Read the model definition and answer for the solid it produces. Units are mm, in the model's axes. A direction names the side the tool comes from. Coordinates: 2 decimals unless noted, no trailing zeros. Loops run counter-clockwise (first coordinate to the right, second up) from the corner with the lowest first, then second, coordinate; pieces in that order, holes last. Notation, with made-up numbers: M 82,-28 L 124,-28 A31 cw 124,10 Z; hole C -40,37 d1. An arc over 180 degrees is marked long. Put each result on its own line as item: value.
from build123d import *

# Parameters (mm, degrees)
F0_R     = 7
F1_DEPTH = 20
F2_R     = 8
F3_DEPTH = 12
F5_DEPTH = 25
F8_DEPTH = 6


with BuildPart() as f1:
    # F0 (on Front) → F1 (new body)
    with BuildSketch(Plane.XZ):
        with BuildLine():
            Line((-35, 54), (-35, 0))
            Line((-35, 0), (35, 0))
            Line((35, 0), (35, 54))
            ThreePointArc((35, 54), (33.242641, 58.242641), (29, 60))
            Line((29, 60), (-29, 60))
            ThreePointArc((-29, 60), (-33.242641, 58.242641), (-35, 54))
        make_face()
        with Locations((-21, 46)):
            Circle(F0_R, mode=Mode.SUBTRACT)
        with Locations((21, 46)):
            Circle(F0_R, mode=Mode.SUBTRACT)
    extrude(amount=F1_DEPTH)

    # F2 (on face) → F3 (join)
    with BuildSketch(Plane(origin=(0, 0, 0), x_dir=(1, 0, 0), z_dir=(0, 0, -1))):
        with BuildLine():
            Line((22, 0), (-22, 0))
            ThreePointArc((-22, 0), (-17.757359, -1.757359), (-16, -6))
            Line((-16, -6), (-16, -80))
            ThreePointArc((-16, -80), (0, -96), (16, -80))
            Line((16, -80), (16, -6))
            ThreePointArc((16, -6), (17.757359, -1.757359), (22, 0))
        make_face()
        with Locations((0, -80)):
            Circle(F2_R, mode=Mode.SUBTRACT)
    extrude(amount=-F3_DEPTH)

    # F7 (on Right) → F8 (join, symmetric)
    with BuildSketch(Plane.YZ):
        with BuildLine():
            Line((0, 12), (30, 12))
            ThreePointArc((30, 12), (8.786797, 20.786797), (0, 42))
            Line((0, 42), (0, 12))
        make_face()
    extrude(amount=F8_DEPTH, both=True)


with BuildPart() as f5:
    # F4 (on Right) → F5 (new body)
    with BuildSketch(Plane.YZ):
        Polygon((8.827168, -95.900685), (44.855885, -95.900685), (44.855885, -23.484161), (8.827168, -23.484161), (8.827168, -49.02795), (8.827168, -76.342739), align=None)
    extrude(amount=F5_DEPTH)


solid = f1.part
1) Find section A-A, the plane z = 46. Write down the section's boundary in (x, y), plus the area to 3 significant figures.
Answer list:
outline: M -35,-20 L -28,-20 L -28,0 L -35,0 Z; M -14,-20 L 14,-20 L 14,0 L -14,0 Z; M 28,-20 L 35,-20 L 35,0 L 28,0 Z
area: 840 mm^2
2) Straight lines are drawn through the part: line 1 (X direction, y = 80, z = 3); line 2 (Z direction, x = 21, y = -9); line 3 (Z direction, x = -8, y = 41.5). For each, find the intervals that lie inside material, in ascending order. Write a range as [from, to].
Answer list:
line 1: x = [-16, -8], [8, 16]
line 2: z = [0, 39], [53, 60]
line 3: z = [0, 12]
3) Given pin 1 Ø2 at (x, y) = (-1, 47.5) entering from +Z; pin 2 Ø18 at (x, z) = (-21, 46) entering from +Y; pin 3 Ø10 at (x, z) = (7, 16.5) entering from +Y; pin 4 Ø12 at (x, y) = (18.5, -2) entering from -Z, each flat-ended and moving along its own axis, determine where each tip first touches the part or whether it passes through.
Answer list:
pin 1: stops at z = 12
pin 2: stops at y = 0
pin 3: stops at y = 95.26
pin 4: stops at z = 0
4) Find section B-B, the plane x = 0. Write down the section's boundary in (y, z).
Answer list:
outline: M -20,0 L 72,0 L 72,12 L 30,12 A30 cw 0,42 L 0,60 L -20,60 Z; M 88,0 L 96,0 L 96,12 L 88,12 Z
5) Find section C-C, the plane y = -13. Write down the section's boundary in (x, z), plus the area to 3 significant figures.
Answer list:
outline: M -35,0 L 35,0 L 35,54 A6 ccw 29,60 L -29,60 A6 ccw -35,54 Z; hole C -21,46 d14; hole C 21,46 d14
area: 3,880 mm^2
6) Determine the mould class of faces 6 (the cylindrical face through (-1.041, 72.068, 5.916)), 7 (the cylindrical face through (33.289, -9.86, 58.196)), 8 (the cylindrical face through (0, 96, 6)) for opening direction Y: released by +Y, released by -Y, zero draft, split by the parting line, or undercut.
Answer list:
face 6: undercut
face 7: zero draft
face 8: released by +Y
7) Find section D-D, the plane z = 18. Write down the section's boundary in (x, y), plus the area to 3 significant figures.
Answer list:
outline: M -35,-20 L 35,-20 L 35,0 L 6,0 L 6,12 L -6,12 L -6,0 L -35,0 Z
area: 1,540 mm^2
8) Which of the six approach directions +Z, -Z, +X, -X, +Y, -Y give full straight-line access (tool end or side, diameter ignored) to faces 1 (the flat face through (-16, 42, 6)), 2 (the flat face through (16, 44, 6)), 3 (the flat face through (-6, 6, 19)), 4 (the flat face through (7, 0, 30)), 5 (the flat face through (6, 6, 19))?
Answer list:
face 1: +Z, -Z, -X, +Y
face 2: +Z, -Z, +X, +Y
face 3: +Z, -X, +Y
face 4: +Z, +Y
face 5: +Z, +X, +Y
